```python
from build123d import *

# Parameters (mm, degrees)
SKETCH_1_W          = 173.4
SKETCH_1_H          = 30
EXTRUDE_1_DEPTH     = 1.25
CHAMFER_1_SIZE      = 8
CHAMFER_2_SIZE      = 2
CUT_EXTRUDE_1_DEPTH = 3.5
CUT_EXTRUDE_4_DEPTH = 3.5
CUT_EXTRUDE_2_DEPTH = 3.5
SKETCH_5_R          = 0.6
CUT_EXTRUDE_3_DEPTH = 3.5
FILLET_1_R          = 0.5
SKETCH_7_W          = 3
SKETCH_7_H          = 5
CUT_EXTRUDE_5_DEPTH = 3.5
SKETCH_8_R          = 0.6
CUT_EXTRUDE_6_DEPTH = 3.5


with BuildPart() as part:
    # 草图1 → 凸台-拉伸1 (new body, symmetric)
    with BuildSketch(Plane.XY):
        with Locations((0, -15)):
            Rectangle(SKETCH_1_W, SKETCH_1_H)
    extrude(amount=EXTRUDE_1_DEPTH, both=True)

    # 倒角1
    chamfer_1_edges = [part.edges().sort_by_distance(p)[0] for p in [
        (86.7, -30, 0),
        (-86.7, -30, 0),
    ]]
    chamfer(chamfer_1_edges, length=CHAMFER_1_SIZE)

    # 倒角2
    chamfer_2_edges = [part.edges().sort_by_distance(p)[0] for p in [
        (-86.7, 0, 0),
        (86.7, 0, 0),
    ]]
    chamfer(chamfer_2_edges, length=CHAMFER_2_SIZE)

    # 草图2 → 切除-拉伸1 (cut, through all)
    with BuildSketch(Plane.XY.offset(1.25)):
        Polygon((-77.2, 0), (-76.2, -2), (-62.2, -2), (-61.2, 0), align=None)
    extrude(amount=-CUT_EXTRUDE_1_DEPTH, mode=Mode.SUBTRACT)

    # 草图6 → 切除-拉伸4 (cut, through all)
    with BuildSketch(Plane.XY.offset(1.25)):
        Polygon((-51.7, 0), (-50.7, -2), (76.2, -2), (77.2, 0), align=None)
    extrude(amount=-CUT_EXTRUDE_4_DEPTH, mode=Mode.SUBTRACT)

    # 草图4 → 切除-拉伸2 (cut, through all)
    with BuildSketch(Plane.XY.offset(1.25)):
        Polygon((-83.325, -2.5), (-79.225, -2.5), (-79.225, -4.5), (-81.225, -4.5), (-81.225, -9.5), (-79.225, -9.5), (-79.225, -11.5), (-83.325, -11.5), align=None)
        Polygon((-59.175, -11.5), (-55.075, -11.5), (-55.075, -2.5), (-59.175, -2.5), (-59.175, -4.5), (-57.175, -4.5), (-57.175, -9.5), (-59.175, -9.5), align=None)
    extrude(amount=-CUT_EXTRUDE_2_DEPTH, mode=Mode.SUBTRACT)

    # 草图5 → 切除-拉伸3 (cut, through all)
    with BuildSketch(Plane.XY.offset(1.25)):
        with Locations((-83.325, -3.1)):
            Circle(SKETCH_5_R)
        with Locations((-83.325, -10.9)):
            Circle(SKETCH_5_R)
        with Locations((-79.825, -11.5)):
            Circle(SKETCH_5_R)
        with Locations((-79.225, -10.1)):
            Circle(SKETCH_5_R)
        with Locations((-79.225, -3.9)):
            Circle(SKETCH_5_R)
        with Locations((-79.825, -2.5)):
            Circle(SKETCH_5_R)
        with Locations((-58.575, -2.5)):
            Circle(SKETCH_5_R)
        with Locations((-59.175, -3.9)):
            Circle(SKETCH_5_R)
        with Locations((-59.175, -10.1)):
            Circle(SKETCH_5_R)
        with Locations((-58.575, -11.5)):
            Circle(SKETCH_5_R)
        with Locations((-55.075, -10.9)):
            Circle(SKETCH_5_R)
        with Locations((-55.075, -3.1)):
            Circle(SKETCH_5_R)
        with Locations((-75.663343685, -1.731671843)):
            Circle(SKETCH_5_R)
        with Locations((-62.736656315, -1.731671843)):
            Circle(SKETCH_5_R)
        with Locations((-50.163343685, -1.731671843)):
            Circle(SKETCH_5_R)
        with Locations((75.663343685, -1.731671843)):
            Circle(SKETCH_5_R)
    extrude(amount=-CUT_EXTRUDE_3_DEPTH, mode=Mode.SUBTRACT)

    # 圆角1
    fillet_1_edges = [part.edges().sort_by_distance(p)[0] for p in [
        (-57.175, -9.5, 0),
        (-57.175, -4.5, 0),
        (-81.225, -4.5, 0),
        (-81.225, -9.5, 0),
    ]]
    fillet(fillet_1_edges, radius=FILLET_1_R)

    # 草图7 → 切除-拉伸5 (cut, through all)
    with BuildSketch(Plane.XY.offset(1.25)):
        with Locations((81.2, -11.5)):
            Rectangle(SKETCH_7_W, SKETCH_7_H)
    extrude(amount=-CUT_EXTRUDE_5_DEPTH, mode=Mode.SUBTRACT)

    # 草图8 → 切除-拉伸6 (cut, through all)
    with BuildSketch(Plane.XY.offset(1.25)):
        with Locations((79.7, -9.6)):
            Circle(SKETCH_8_R)
        with Locations((79.7, -13.4)):
            Circle(SKETCH_8_R)
        with Locations((82.7, -13.4)):
            Circle(SKETCH_8_R)
        with Locations((82.7, -9.6)):
            Circle(SKETCH_8_R)
    extrude(amount=-CUT_EXTRUDE_6_DEPTH, mode=Mode.SUBTRACT)


solid = part.part
```
CAD build for the part. Positions are in the model's coordinates, mm. Round coordinates to 2 decimals unless told otherwise and drop trailing zeros. Write each loop counter-clockwise with the first axis right and the second up, starting at its lowest first coordinate (ties: lowest second). Pieces come first, ordered by that corner, then holes.
Item 1: Band-saw the part on D-D on x = -16. Write the cut outline in (y, z), then the cut area to 3 significant figures.
Filled in:
outline: (-30, -1.25) - (-2, -1.25) - (-2, 1.25) - (-30, 1.25) - close
area: 70.0 mm2
Item 2: Band-saw the part on C-C on y = -23.5. Write the cut outline in (x, z), then the cut area to 3 significant figures.
Filled in:
outline: (-85.2, -1.25) - (85.2, -1.25) - (85.2, 1.25) - (-85.2, 1.25) - close
area: 426 mm2
Item 3: Band-saw the part on A-A on y = -7.5. Write the cut outline in (x, z) (3 decimals), then the cut area to 3 significant figures.
Filled in:
outline: (-86.7, -1.25) - (-83.325, -1.25) - (-83.325, 1.25) - (-86.7, 1.25) - close; (-81.225, -1.25) - (-57.175, -1.25) - (-57.175, 1.25) - (-81.225, 1.25) - close; (-55.075, -1.25) - (86.7, -1.25) - (86.7, 1.25) - (-55.075, 1.25) - close
area: 423 mm2
Item 4: Drill centre lines: L1, parallel to X at y = -5, z = 0.75 (3 decimals); L2, parallel to Y at x = -32, z = 0.55; L3, parallel to X at y = -24.5, z = -0.35. Where is each one in solid material? Low to high.
Filled in:
L1: x = -86.7 to -83.325, -81.225 to -57.175, -55.075 to 86.7
L2: y = -30 to -2
L3: x = -84.2 to 84.2
Item 5: Drop flat-ended pins along their axis: pin 1 Ø1.2 at (x, z) = (81, -0.5) entering from -Y; pin 2 Ø1.2 at (x, z) = (18, -0.5) entering from +Y. Give the stop position or say it passes through.
Filled in:
pin 1: stops at y = -28.3
pin 2: stops at y = -2
Item 6: Band-saw the part on B-B on z = -0.4. Give the number of separate pieces and of enclosed holes in the cut face, then the cut area to 3 significant figures.
Filled in:
separate pieces: 1
enclosed holes: 3
area: 4,770 mm2
